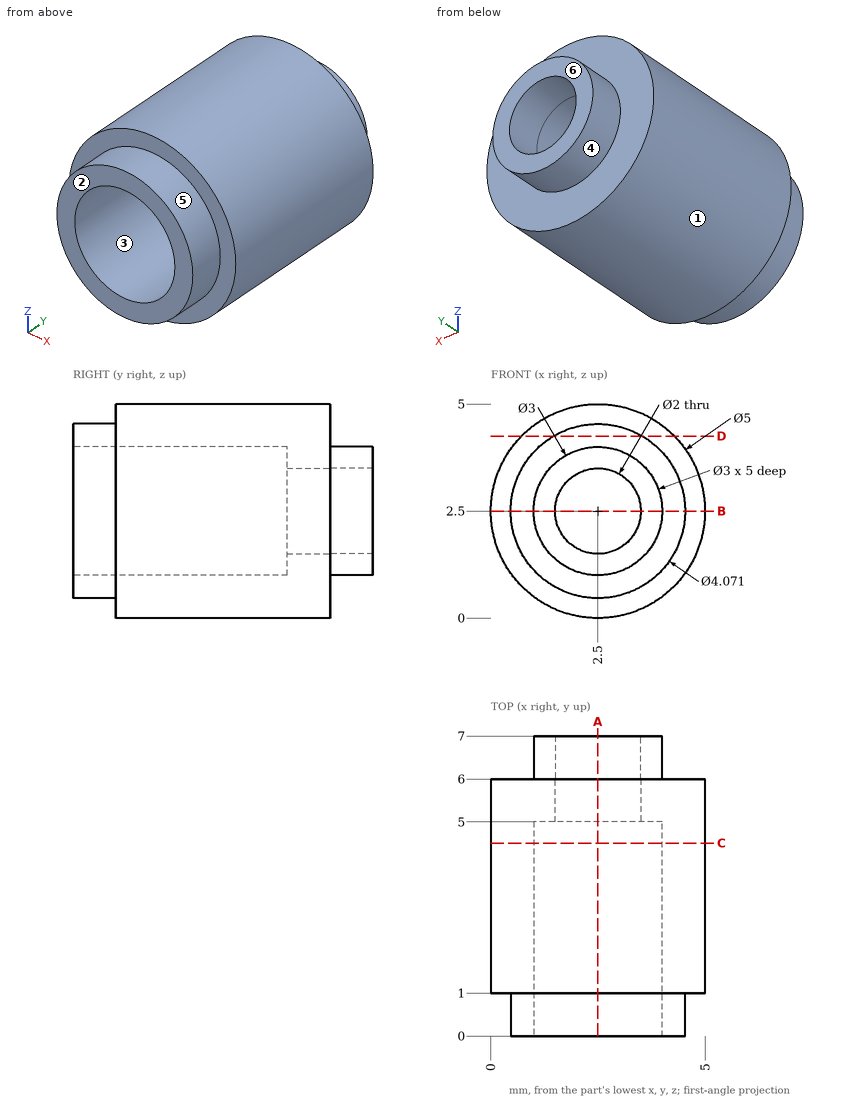
Could you check a few things on this drawing? It's one solid part, dimensions in mm from its lowest x, y, z. A direction names the side the tool comes from. Give positions to 0.01 mm unless a question says otherwise; leave off trailing zeros. Order: outer loops, then holes, each group sorted by start corner. A loop starts at its lowest first (then second) coordinate and runs counter-clockwise, first axis right, second up. Notation, with made-up numbers: (-28, 29) -> (25, 29) arc R15 ccw to (25, 47) -> close; hole circle Ø5 at (15, 8.5). An arc over 180 degrees is marked (long way). Answer in a Markdown table with one row per item. Add a question column.
Item 1: Imagine slicing it at A-A (x = 2.5). List the corners of the cut face in (y, z) for me, and give its area (3 significant figures).
Item 2: Imagine slicing it at C-C (y = 4.5). List the corners of the cut face in (x, z) for me.
Item 3: We'd pull the mould along Z, two halves only. Please class the marked faces 1, 2 and 3: pulls with the +Z half, pulls with the -Z half, needs draft (parallel to the pull), parting line crosses it, or undercut.
Item 4: I'm going to push flat-ended pins straight in: P1, Ø3, axis at x = 2, y = 4.5, coming from the -Z side; P2, Ø1, axis at x = 1.5, y = 1.5, coming from the +Z side; P3, Ø1, axis at x = 1.5, z = 4.5, coming from the +Y side. Where does each tip first touch, or does it pass through?
Item 5: For the marked faces 4, 5 and 6, which set-ups out of +Z, -Z, +X, -X, +Y, -Y let a thin tool reach every point of the face, with its end or its side?
Item 6: Imagine slicing it at B-B (z = 2.5). List the corners of the cut face in (x, y) for me.
Item 7: Imagine slicing it at D-D (z = 4.25). List the corners of the cut face in (x, y) for me.
Item 8: Please list where these lines run through material, in increasing order: probe 1 along X at (y, z) = (2.15, 2.5); probe 2 along X at (y, z) = (6.5, 2.5).
Result:
| question | item | result |
|---|---|---|
| 1 | outline | (0, 0.46) -> (1, 0.46) -> (1, 0) -> (6, 0) -> (6, 1) -> (7, 1) -> (7, 1.5) -> (5, 1.5) -> (5, 1) -> (0, 1) -> close; (0, 4) -> (5, 4) -> (5, 3.5) -> (7, 3.5) -> (7, 4) -> (6, 4) -> (6, 5) -> (1, 5) -> (1, 4.54) -> (0, 4.54) -> close |
| 1 | area | 13.1 mm2 |
| 2 | outline | circle Ø5 at (2.5, 2.5); hole circle Ø3 at (2.5, 2.5) |
| 3 | face 1 | parting line crosses it |
| 3 | face 2 | needs draft |
| 3 | face 3 | undercut |
| 4 | P1 | z = 0 |
| 4 | P2 | z = 4.95 |
| 4 | P3 | y = 6 |
| 5 | face 4 | +Y |
| 5 | face 5 | -Y |
| 5 | face 6 | +Z, -Z, +X, -X, +Y |
| 6 | outline | (0, 1) -> (0.46, 1) -> (0.46, 0) -> (1, 0) -> (1, 5) -> (1.5, 5) -> (1.5, 7) -> (1, 7) -> (1, 6) -> (0, 6) -> close; (3.5, 5) -> (4, 5) -> (4, 0) -> (4.54, 0) -> (4.54, 1) -> (5, 1) -> (5, 6) -> (4, 6) -> (4, 7) -> (3.5, 7) -> close |
| 7 | outline | (0.71, 1) -> (1.46, 1) -> (1.46, 0) -> (3.54, 0) -> (3.54, 1) -> (4.29, 1) -> (4.29, 6) -> (0.71, 6) -> close |
| 8 | probe 1 | 0 to 1, 4 to 5 |
| 8 | probe 2 | 1 to 1.5, 3.5 to 4 |
